```python
from build123d import *

# Parameters (mm, degrees)
F1_DEPTH = 3.175
F2_R     = 4.3688
F2_R_2   = 25.4
F3_DEPTH = 6.351


with BuildPart() as f1:
    # F0 (on Front) → F1 (new body, symmetric)
    with BuildSketch(Plane.XZ):
        Polygon((98.933, 0), (-98.933, 0), (-244.983, -146.05), (244.983, -146.05), align=None)
    extrude(amount=F1_DEPTH, both=True)

    # F2 (on face) → F3 (cut, through all)
    with BuildSketch(Plane.XZ.offset(3.175)):
        with Locations((67.437, -76.2)):
            Circle(F2_R)
        with Locations((67.437, -120.65)):
            Circle(F2_R)
        with Locations((-67.437, -76.2)):
            Circle(F2_R)
        with Locations((-67.437, -120.65)):
            Circle(F2_R)
        with Locations((-118.237, -98.425)):
            Circle(F2_R_2)
        with Locations((118.237, -98.425)):
            Circle(F2_R_2)
    extrude(amount=-F3_DEPTH, mode=Mode.SUBTRACT)


solid = f1.part
```
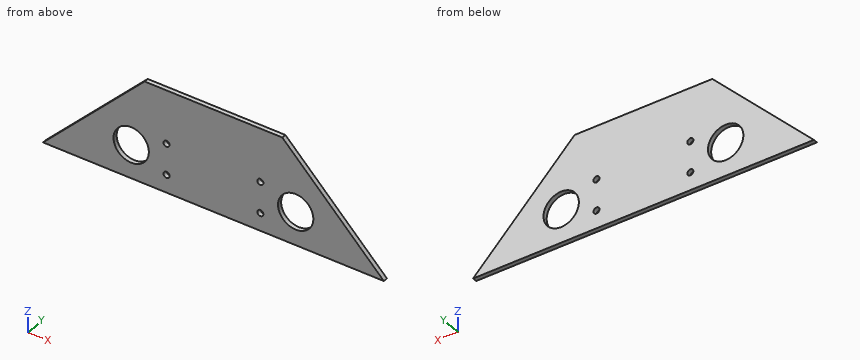
The model under review builds one solid part; all positions refer to its coordinate system, in mm. Round coordinates to 2 decimals unless told otherwise and drop trailing zeros. Order: outer loops, then holes, each group sorted by start corner. A loop starts at its lowest first (then second) coordinate and runs counter-clockwise, first axis right, second up. Notation, with made-up numbers: (11, 46.25) - (68, 46.25) arc R14 ccw to (68, 55.25) - close; hole circle Ø2 at (-12, 75). An arc over 180 degrees is marked (long way). Answer in a Markdown table with one row per item.
(1) Clearance check with a flat-ended pin moving along its axis: P1, Ø2, axis at y = 0, z = -82, coming from the -X side. State where the tip first meets the part, or that it passes through.
Result set:
| item | result |
|---|---|
| P1 | stops at x = -181.93 |
(2) Take a section at B-B on z = -46.5. Write out the cut boundary in (x, y) (3 decimals).
Result set:
| item | result |
|---|---|
| outline | (-145.433, -3.175) - (145.433, -3.175) - (145.433, 3.175) - (-145.433, 3.175) - close |
(3) For line 1 (X direction, y = 0.5, z = -84); line 2 (X direction, y = -2.25, z = -89); line 3 (Z direction, x = 112.5, y = -1.75), list the stretches that pass through material, from the lowest coordinate up. Write a range as from..to.
Result set:
| item | result |
|---|---|
| line 1 | x = -182.93..-139.14, -97.33..97.33, 139.14..182.93 |
| line 2 | x = -187.93..-141.82, -94.65..94.65, 141.82..187.93 |
| line 3 | z = -146.05..-123.17, -73.68..-13.57 |
(4) Take a section at C-C on z = -20. Write out the cut boundary in (x, y) (3 decimals).
Result set:
| item | result |
|---|---|
| outline | (-118.933, -3.175) - (118.933, -3.175) - (118.933, 3.175) - (-118.933, 3.175) - close |
(5) Take a section at A-A on y = 0.5. Write out the cut boundary in (x, z) (3 decimals), plus the area to 3 significant figures.
Result set:
| item | result |
|---|---|
| outline | (-244.983, -146.05) - (244.983, -146.05) - (98.933, 0) - (-98.933, 0) - close; hole circle Ø50.8 at (-118.237, -98.425); hole circle Ø8.738 at (-67.437, -120.65); hole circle Ø8.738 at (-67.437, -76.2); hole circle Ø8.738 at (67.437, -120.65); hole circle Ø8.738 at (67.437, -76.2); hole circle Ø50.8 at (118.237, -98.425) |
| area | 45,900 mm2 |
